Geometry check sheet. Reference: the model listing, model coordinates, mm. Face numbers are marked on the shaded views. A direction names the side the tool comes from. Round coordinates to 2 decimals unless told otherwise and drop trailing zeros. Loops run counter-clockwise (first coordinate to the right, second up) from the corner with the lowest first, then second, coordinate; pieces in that order, holes last.
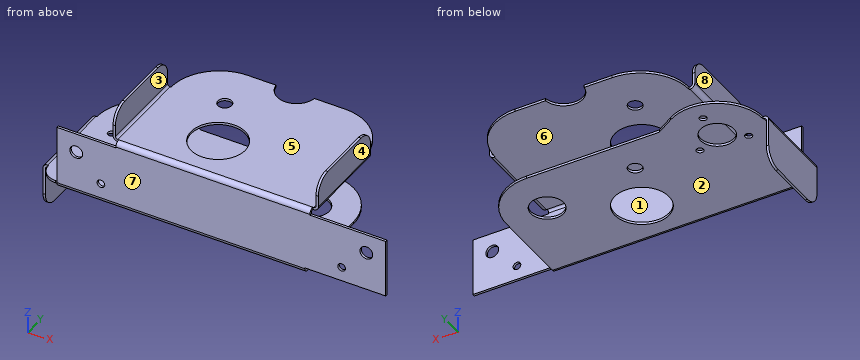
```python
from build123d import *

# Parameters (mm, degrees)
SKETCH1_W                = 101.6
SKETCH1_H                = 18
BASE_FLANGE1_DEPTH       = 0.7366
CUT_EXTRUDE1_DEPTH       = 248.362817644
CUT_EXTRUDE1_DEPTH_BACK  = 248.362817644
SKETCH9_R                = 1.984375
SKETCH9_R_2              = 1.190625
EDGE_FLANGE2_DEPTH       = 60
CUT_EXTRUDE10_DEPTH      = 276.770749451
CUT_EXTRUDE10_DEPTH_BACK = 276.770749451
SKETCH47_R               = 5.065
SKETCH48_R               = 6
CUT_EXTRUDE11_DEPTH      = 10
EDGE_FLANGE4_DEPTH       = 76.6
EDGE_FLANGE4_START       = 0.7366
EDGE_FLANGE4_FLAT_DEPTH  = 0.7366
CUT_EXTRUDE12_DEPTH      = 105.880550385
CUT_EXTRUDE12_DEPTH_BACK = 105.880550385
SKETCH52_R               = 2.15
TAB1_START               = -0.7366
TAB1_OUTLINE_W           = 10
TAB1_OUTLINE_H           = 49.408594005
TAB1_DEPTH               = 0.7366
SKETCH56_R               = 5.065
CUT_EXTRUDE13_DEPTH      = 5
CUT_EXTRUDE16_DEPTH      = 105.732220975
CUT_EXTRUDE16_DEPTH_BACK = 105.732220975
SKETCH59_R               = 1.1
SKETCH59_R_2             = 5.17
CUT_EXTRUDE18_DEPTH      = 10
FILLET1_R                = 5
EDGE_FLANGE5_DEPTH       = 25.419820015
FILLET2_R                = 5
FILLET3_R                = 15
EDGE_FLANGE6_DEPTH       = 27.460964596
EDGE_FLANGE6_BEND_DEPTH  = 27.460964596
FILLET4_R                = 5
SKETCH71_R               = 8.39617584
CUT_EXTRUDE19_DEPTH      = 83.479179892


# Read off the part's stored shape, not the designer's step: Tab1
# Sheet-metal steps are written as plain solids
with BuildPart() as part:
    # Sketch1 → Base-Flange1 (new body)
    with BuildSketch(Plane(origin=(0, 0, 0), x_dir=(1, 0, 0), z_dir=(0, 1, 0))):
        Rectangle(SKETCH1_W, SKETCH1_H)
    extrude(amount=-BASE_FLANGE1_DEPTH)

    # Sketch9 → Cut-Extrude1 (cut, two sides: drawn at the far end of the back side and taken through both)
    with BuildSketch(Plane(origin=(-165.711822879, -0.7366, -110.626299478), x_dir=(0.7071067811865437, 0, -0.7071067811865515), z_dir=(0, 1, 0)).offset(-CUT_EXTRUDE1_DEPTH_BACK)):
        with Locations(Location((5.089841868, -165.843496765, 0), (0, 0, 135))):
            Circle(SKETCH9_R)
        with Locations(Location((15.884109726, -165.843496765, 0), (0, 0, 135))):
            Circle(SKETCH9_R_2)
        with Locations(Location((68.508410595, -229.262065492, 0), (0, 0, 135))):
            Circle(SKETCH9_R)
        with Locations(Location((68.508410595, -218.467797635, 0), (0, 0, 135))):
            Circle(SKETCH9_R_2)
    extrude(amount=CUT_EXTRUDE1_DEPTH + CUT_EXTRUDE1_DEPTH_BACK, mode=Mode.SUBTRACT)

    # Edge-Flange2 section (across the edge) → Edge-Flange2 (add)
    with BuildSketch(Plane(origin=(-32.583570882, 0, 10), x_dir=(0, 0, -1), z_dir=(1, 0, 0))):
        with BuildLine():
            Line((-0.7366, 0.7366), (-0.7366, 43.197564596))
            Line((-0.7366, 43.197564596), (0, 43.197564596))
            Line((0, 43.197564596), (0, 0.7366))
            ThreePointArc((0, 0.7366), (0.215745145, 0.215745145), (0.7366, 0))
            Line((0.7366, 0), (1, 0))
            Line((1, 0), (1, -0.7366))
            Line((1, -0.7366), (0.7366, -0.7366))
            ThreePointArc((0.7366, -0.7366), (-0.30510971, -0.30510971), (-0.7366, 0.7366))
        make_face()
    extrude(amount=EDGE_FLANGE2_DEPTH)

    # Sketch47 → Cut-Extrude10 (cut, two sides: drawn at the far end of the back side and taken through both)
    with BuildSketch(Plane(origin=(-165.711822879, -125.530580752, -15.7766), x_dir=(1, 0, 0), z_dir=(0, 0, 1)).offset(-CUT_EXTRUDE10_DEPTH_BACK)):
        with Locations((162.765212711, 169.489973714)):
            Circle(SKETCH47_R)
    extrude(amount=CUT_EXTRUDE10_DEPTH + CUT_EXTRUDE10_DEPTH_BACK, mode=Mode.SUBTRACT)

    # Sketch48 → Cut-Extrude11 (cut)
    with BuildSketch(Plane.XY.offset(10.7366)):
        with Locations((-2.946610168, 43.959392962)):
            Circle(SKETCH48_R)
    extrude(amount=-CUT_EXTRUDE11_DEPTH, mode=Mode.SUBTRACT)

    # Edge-Flange4 bend section (across the edge) → Edge-Flange4 (add)
    with BuildSketch(Plane(origin=(25.8, 0, -10), x_dir=(0, 0, 1), z_dir=(-1, 0, 0))):
        with BuildLine():
            Line((-0.7366, 0.7366), (0, 0.7366))
            ThreePointArc((0, 0.7366), (0.215745145, 0.215745145), (0.7366, 0))
            Line((0.7366, 0), (1, 0))
            Line((1, 0), (1, -0.7366))
            Line((1, -0.7366), (0.7366, -0.7366))
            ThreePointArc((0.7366, -0.7366), (-0.30510971, -0.30510971), (-0.7366, 0.7366))
        make_face()
    extrude(amount=EDGE_FLANGE4_DEPTH)

    # Edge-Flange4 profile (on flange) → Edge-Flange4 flat (add)
    with BuildSketch(Plane(origin=(0, 0, -10), x_dir=(-1, 0, 0), z_dir=(0, 0, -1)).offset(EDGE_FLANGE4_START)):
        Polygon((-25.8, 40), (-25.8, 0.7366), (50.8, 0.7366), (50.8, 40), (50.8, 50.145194005), (30.27574847, 50.145194005), (30.27574847, 40), align=None)
    extrude(amount=-EDGE_FLANGE4_FLAT_DEPTH)

    # Sketch52 → Cut-Extrude12 (cut, two sides: drawn at the far end of the back side and taken through both)
    with BuildSketch(Plane(origin=(-25.053389833, -19.029185513, -10.7366), x_dir=(-1, 0, 0), z_dir=(0, 0, -1)).offset(-CUT_EXTRUDE12_DEPTH_BACK)):
        with Locations(Location((-8.524599638, 48.296752149, 0), (0, 0, 90))):
            Circle(SKETCH52_R)
    extrude(amount=CUT_EXTRUDE12_DEPTH + CUT_EXTRUDE12_DEPTH_BACK, mode=Mode.SUBTRACT)

    # Tab1 outline → Tab1 (add)
    with BuildSketch(Plane.XY.offset(-10).offset(TAB1_START)):
        with Locations((-55.8, 25.440897003)):
            Rectangle(TAB1_OUTLINE_W, TAB1_OUTLINE_H)
    extrude(amount=TAB1_DEPTH)

    # Sketch56 → Cut-Extrude13 (cut)
    with BuildSketch(Plane(origin=(-25.053389833, -19.029185513, -11.4732), x_dir=(-1, 0, 0), z_dir=(0, 0, -1))):
        with Locations(Location((-37.853389832, 44.695992962, 0), (0, 0, 90))):
            Circle(SKETCH56_R)
    extrude(amount=-CUT_EXTRUDE13_DEPTH, mode=Mode.SUBTRACT)

    # Sketch59 → Cut-Extrude16 (cut, two sides: drawn at the far end of the back side and taken through both)
    with BuildSketch(Plane(origin=(-25.053389833, -19.029185513, -10), x_dir=(1, 0, 0), z_dir=(0, 0, 1)).offset(-CUT_EXTRUDE16_DEPTH_BACK)):
        with Locations(Location((-24.955394773, 45.581923383, 0), (0, 0, 180))):
            Circle(SKETCH59_R)
        with Locations(Location((-17.957123001, 50.185605529, 0), (0, 0, 180))):
            Circle(SKETCH59_R_2)
        with Locations(Location((-18.462707804, 58.547069581, 0), (0, 0, 180))):
            Circle(SKETCH59_R)
        with Locations(Location((-10.455133223, 46.458697096, 0), (0, 0, 180))):
            Circle(SKETCH59_R)
    extrude(amount=CUT_EXTRUDE16_DEPTH + CUT_EXTRUDE16_DEPTH_BACK, mode=Mode.SUBTRACT)

    # Sketch61 → Cut-Extrude18 (cut)
    with BuildSketch(Plane.XY.offset(-10)):
        with BuildLine():
            Line((-57.180512833, 31.156420015), (-57.180512833, 0.7366))
            Line((-57.180512833, 0.7366), (-60.8, 0.7366))
            Line((-60.8, 0.7366), (-60.8, 50.145194005))
            Line((-60.8, 50.145194005), (-30.27574847, 50.145194005))
            Line((-30.27574847, 50.145194005), (-30.27574847, 40))
            Line((-30.27574847, 40), (-35.653602425, 43.266943094))
            ThreePointArc((-35.653602425, 43.266943094), (-49.958227548, 43.506244316), (-57.180512833, 31.156420015))
        make_face()
    extrude(amount=-CUT_EXTRUDE18_DEPTH, mode=Mode.SUBTRACT)

    # Fillet1
    fillet1_edges = [part.edges().sort_by_distance(p)[0] for p in [
        (-57.180512833, 0.7366, -10.3683),
    ]]
    fillet(fillet1_edges, radius=FILLET1_R)

    # Edge-Flange5 section (across the edge) → Edge-Flange5 (add)
    with BuildSketch(Plane(origin=(-58.180512833, 5.7366, -10.7366), x_dir=(1, 0, 0), z_dir=(0, 1, 0))):
        with BuildLine():
            Line((-0.7366, 0.7366), (-0.7366, 14.2634))
            Line((-0.7366, 14.2634), (0, 14.2634))
            Line((0, 14.2634), (0, 0.7366))
            ThreePointArc((0, 0.7366), (0.215745145, 0.215745145), (0.7366, 0))
            Line((0.7366, 0), (1, 0))
            Line((1, 0), (1, -0.7366))
            Line((1, -0.7366), (0.7366, -0.7366))
            ThreePointArc((0.7366, -0.7366), (-0.30510971, -0.30510971), (-0.7366, 0.7366))
        make_face()
    extrude(amount=EDGE_FLANGE5_DEPTH)

    # Fillet2
    fillet2_edges = [part.edges().sort_by_distance(p)[0] for p in [
        (-58.548812833, 5.7366, -25),
        (-58.548812833, 31.156420015, -25),
    ]]
    fillet(fillet2_edges, radius=FILLET2_R)

    # Fillet3
    fillet3_edges = [part.edges().sort_by_distance(p)[0] for p in [
        (25.8, 40, -10.3683),
        (-32.583570882, 43.197564596, 10.3683),
        (27.416429118, 43.197564596, 10.3683),
    ]]
    fillet(fillet3_edges, radius=FILLET3_R)

    # Edge-Flange6 section (across the edge) → Edge-Flange6 (add)
    with BuildSketch(Plane(origin=(28.416429118, 0.7366, 10.7366), x_dir=(-1, 0, 0), z_dir=(0, 1, 0))):
        with BuildLine():
            Line((-0.7366, 0.7366), (-0.7366, 9.2634))
            Line((-0.7366, 9.2634), (0, 9.2634))
            Line((0, 9.2634), (0, 0.7366))
            ThreePointArc((0, 0.7366), (0.215745145, 0.215745145), (0.7366, 0))
            Line((0.7366, 0), (1, 0))
            Line((1, 0), (1, -0.7366))
            Line((1, -0.7366), (0.7366, -0.7366))
            ThreePointArc((0.7366, -0.7366), (-0.30510971, -0.30510971), (-0.7366, 0.7366))
        make_face()
    extrude(amount=EDGE_FLANGE6_DEPTH)

    # Edge-Flange6 section 2 (across the edge) → Edge-Flange6 bend (add)
    with BuildSketch(Plane(origin=(-33.583570882, 28.197564596, 10.7366), x_dir=(1, 0, 0), z_dir=(0, -1, 0))):
        with BuildLine():
            Line((-0.7366, 0.7366), (-0.7366, 9.2634))
            Line((-0.7366, 9.2634), (0, 9.2634))
            Line((0, 9.2634), (0, 0.7366))
            ThreePointArc((0, 0.7366), (0.215745145, 0.215745145), (0.7366, 0))
            Line((0.7366, 0), (1, 0))
            Line((1, 0), (1, -0.7366))
            Line((1, -0.7366), (0.7366, -0.7366))
            ThreePointArc((0.7366, -0.7366), (-0.30510971, -0.30510971), (-0.7366, 0.7366))
        make_face()
    extrude(amount=EDGE_FLANGE6_BEND_DEPTH)

    # Fillet4
    fillet4_edges = [part.edges().sort_by_distance(p)[0] for p in [
        (28.784729118, 0.7366, 20),
        (28.784729118, 28.197564596, 20),
        (-33.951870882, 28.197564596, 20),
        (-33.951870882, 0.7366, 20),
    ]]
    fillet(fillet4_edges, radius=FILLET4_R)

    # Sketch71 → Cut-Extrude19 (cut, through all)
    with BuildSketch(Plane.XY.offset(10.7366)):
        with Locations((-9.454494987, 13.710785706)):
            Circle(SKETCH71_R)
    extrude(amount=-CUT_EXTRUDE19_DEPTH, mode=Mode.SUBTRACT)


solid = part.part
```
1) Sectioned sample at D-D, the plane x = 41.5. Record the cut outline in (y, z), then the cut area to 3 significant figures.
Report:
outline: (-0.74, -9) - (0, -9) - (0, 9) - (-0.74, 9) - close
area: 13.3 mm2
2) Gauge pin test, flat ends, axial feed: pin 1 (0.7 mm diameter, centred on y = 0, z = -4.5, fed in from -X); pin 2 (4 mm diameter, centred on x = 4, y = 18, fed in from +Z); pin 3 (1.5 mm diameter, centred on x = 6.5, y = 10, fed in from -Z); pin 4 (1.4 mm diameter, centred on x = -37.211, z = -4.589, fed in from -Y). Record the tip position at first contact, or that the pin passes through.
Report:
pin 1: stops at x = -50.8
pin 2: stops at z = 10.74
pin 3: stops at z = -10.74
pin 4: passes through
3) Sectioned sample at B-B, the plane x = -12. Record the cut outline in (y, z).
Report:
outline: (-0.74, -9.26) arc R1.47 ccw to (0.74, -10.74) - (5.71, -10.74) - (5.71, -10) - (0.74, -10) arc R0.74 cw to (0, -9.26) - (0, 9.26) arc R0.74 cw to (0.74, 10) - (5.71, 10) - (5.71, 10.74) - (0.74, 10.74) arc R1.47 ccw to (-0.74, 9.26) - close; (21.71, -10.74) - (40, -10.74) - (40, -10) - (21.71, -10) - close; (21.71, 10) - (43.2, 10) - (43.2, 10.74) - (21.71, 10.74) - close
4) Access from +Z, -Z, +X, -X, +Y, -Y to the whole of each face (thin tool, end or side, straight path). Record for the marked faces 4, 5, 6, 7 and 8.
Report:
face 4: +Z, -Z, +X, +Y, -Y
face 5: +Z, +Y, -Y
face 6: +X, -X, +Y
face 7: +Z, -Z, +X, -X, -Y
face 8: +Z, -X, +Y, -Y
5) Sectioned sample at A-A, the plane y = 15.5. Record the cut outline in (x, z), then the cut area to 3 significant figures.
Report:
outline: (-58.92, -25) - (-58.18, -25) - (-58.18, -11.47) arc R0.74 cw to (-57.44, -10.74) - (-17.66, -10.74) - (-17.66, -10) - (-57.44, -10) arc R1.47 ccw to (-58.92, -11.47) - close; (-34.32, 11.47) arc R1.47 ccw to (-32.85, 10) - (-17.66, 10) - (-17.66, 10.74) - (-32.85, 10.74) arc R0.74 cw to (-33.58, 11.47) - (-33.58, 20) - (-34.32, 20) - close; (-1.25, -10.74) - (25.8, -10.74) - (25.8, -10) - (-1.25, -10) - close; (-1.25, 10) - (27.68, 10) arc R1.47 ccw to (29.15, 11.47) - (29.15, 20) - (28.42, 20) - (28.42, 11.47) arc R0.74 cw to (27.68, 10.74) - (-1.25, 10.74) - close
area: 108 mm2
6) Mould release check, pull along Z, two halves, no side actions. Record for the marked faces 1, 2 and 3: +Z half, -Z half, draft (parallel to the pull), parting line (faces both ways), or undercut.
Report:
face 1: undercut
face 2: -Z half
face 3: draft
7) Scan lines: line 1 along Z through (x, y) = (-15, 25.5); line 2 along Y through (x, z) = (-39, 5); line 3 along Z through (x, y) = (-46.5, 25). Record each from-to range of solid material in increasing order.
Report:
line 1: z = -10.74 to -10, 10 to 10.74
line 2: y = -0.74 to 0
line 3: z = -10.74 to -10
8) Sectioned sample at C-C, the plane x = -29. Record the cut outline in (y, z), then the cut area to 3 significant figures.
Report:
outline: (-0.74, -9.26) arc R1.47 ccw to (0.74, -10.74) - (40, -10.74) - (40, -10) - (0.74, -10) arc R0.74 cw to (0, -9.26) - (0, 9.26) arc R0.74 cw to (0.74, 10) - (37.93, 10) - (37.93, 10.74) - (0.74, 10.74) arc R1.47 ccw to (-0.74, 9.26) - close
area: 72.5 mm2
